The drawing under review shows one solid part. Ordinate dimensions are in mm from its lowest x, y, z. Give positions to 0.01 mm unless a question says otherwise; leave off trailing zeros. Loops run counter-clockwise (first coordinate to the right, second up) from the corner with the lowest first, then second, coordinate; pieces in that order, holes last. Notation, with made-up numbers: M 23,-19.75 L 66,-19.75 A25 ccw 66,-2.75 Z; hole C 22.5,79 d7. An arc over 180 degrees is marked long. Put each result on its own line as item: value. Start each with the question number.
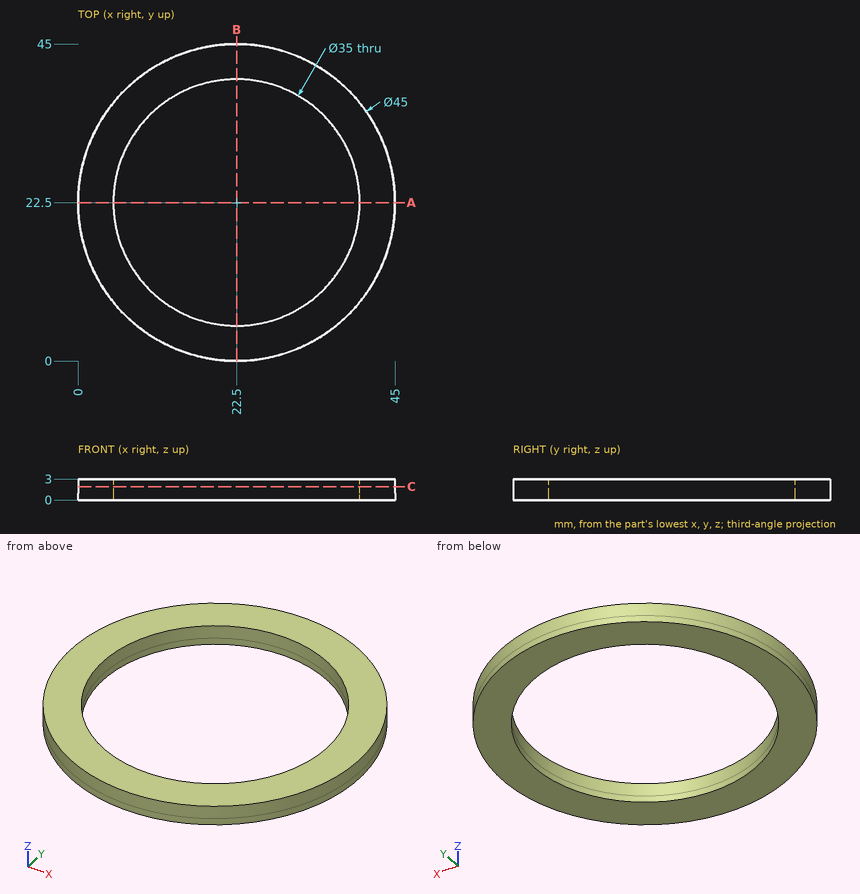
(1) To check wall thickness, follow L1, parallel to Y at x = 22.5, z = 0.25; L2, parallel to X at y = 27, z = 1.25; L3, parallel to Y at x = 34.5, z = 1.35. State the ranges of each line that lie inside material, in increasing order. Write a range as [from, to].
(2) We need section A-A, the plane y = 22.5. Write out the cut boundary in (x, z).
(3) We need section C-C, the plane z = 1.9. Write out the cut boundary in (x, y).
(4) Insertion check: pin 1 (1 mm diameter, centred on y = 30.5, z = 2, fed in from -X); pin 2 (1 mm diameter, centred on x = 10.5, z = 1, fed in from +Y). Each pin has a flat end and moves straight along its axis. Give the tip position at first contact, or say it passes through.
Check sheet entries:
1. L1: y = [0, 5], [40, 45]
1. L2: x = [0.45, 5.59], [39.41, 44.55]
1. L3: y = [3.47, 9.76], [35.24, 41.53]
2. outline: M 0,0 L 5,0 L 5,3 L 0,3 Z; M 40,0 L 45,0 L 45,3 L 40,3 Z
3. outline: C 22.5,22.5 d45; hole C 22.5,22.5 d35
4. pin 1: stops at x = 1.29
4. pin 2: stops at y = 41.84
